The drawing under review shows one solid part. Ordinate dimensions are in mm from its lowest x, y, z. A direction names the side the tool comes from. Coordinates: 2 decimals unless noted, no trailing zeros. Write each loop counter-clockwise with the first axis right and the second up, starting at its lowest first coordinate (ties: lowest second). Pieces come first, ordered by that corner, then holes.
Q1. Machinability: for the marked faces 1, 2 and 3, which of the approach directions +Z, -Z, +X, -X, +Y, -Y give a long, thin tool a straight path to every point of the face, cutting with its end or side? Answer none if there is none.
Q2. Mouldability with a two-part tool opening along Z and no side actions: class the marked faces 4, 5, 6 and 7 as pulls with the +Z half, pulls with the -Z half, needs draft (parallel to the pull), parting line crosses it, or undercut.
Q3. For probe 1 along Z at (x, y) = (825, 170); probe 2 along Z at (x, y) = (845, 150.5); probe 3 along Z at (x, y) = (438, 390.5), list the stretches that pass through material, from the lowest coordinate up.
Q4. Take a section at A-A (y = 136.5). Give the boundary of the cut face in (x, z), and give its area (3 significant figures).
Q5. Insertion check: pin 1 (1 mm diameter, centred on y = 300, z = 417, fed in from +X); pin 2 (12 mm diameter, centred on y = 62.5, z = 791.5, fed in from +X) (1 decimal); pin 3 (10 mm diameter, centred on y = 73.5, z = 890.5, fed in from +X). Each pin has a flat end and moves straight along its axis. Give the tip position at first contact, or say it passes through.
Q6. Take a section at C-C (z = 243.5). Give the boundary of the cut face in (x, y) (1 decimal).
Q7. Take a section at B-B (x = 825.5). Give the boundary of the cut face in (y, z).
Q8. Take a section at D-D (x = 1266). Give the boundary of the cut face in (y, z).
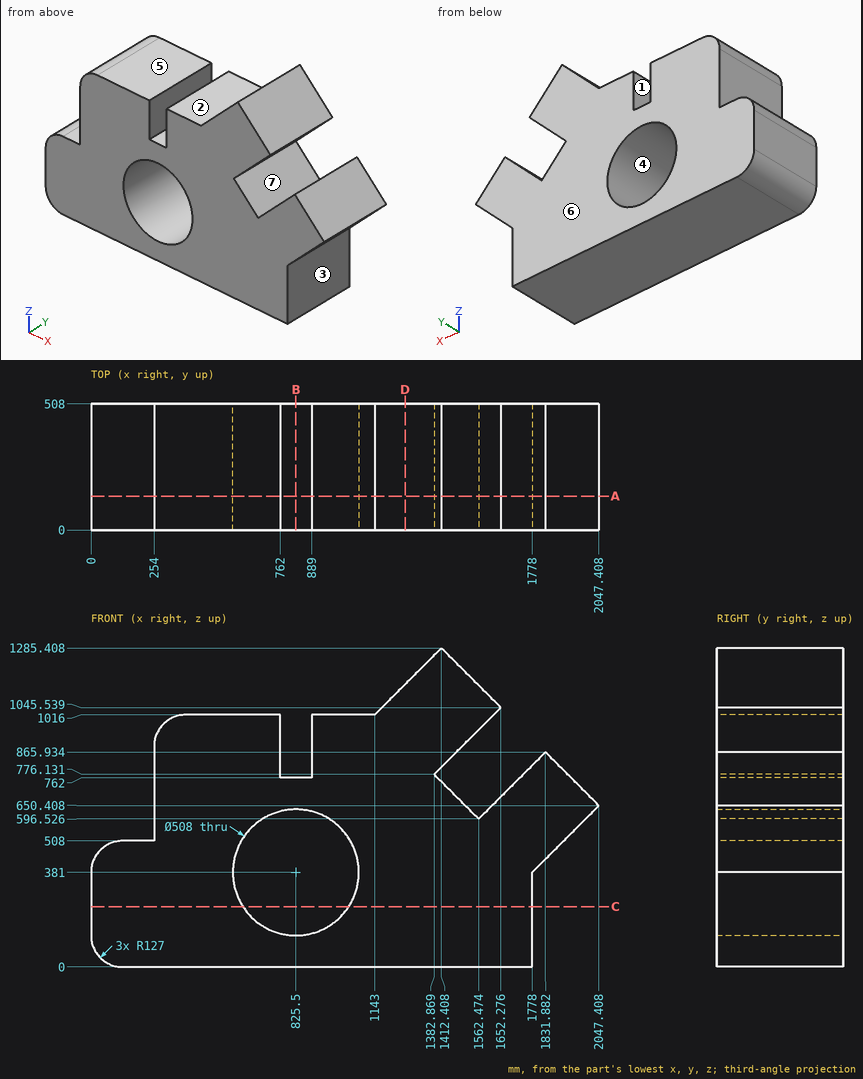
Response:
1. face 1: +Z, +Y, -Y
1. face 2: +Z, -X, +Y, -Y
1. face 3: -Z, +X, +Y, -Y
2. face 4: undercut
2. face 5: pulls with the +Z half
2. face 6: needs draft
2. face 7: undercut
3. probe 1: z = 0 to 127, 635 to 762
3. probe 2: z = 0 to 127.75, 634.25 to 762
3. probe 3: z = 0 to 1016
4. outline: (0, 127) arc R127 ccw to (127, 0) - (1778, 0) - (1778, 381) - (2047.41, 650.41) - (1831.88, 865.93) - (1562.47, 596.53) - (1382.87, 776.13) - (1652.28, 1045.54) - (1412.41, 1285.41) - (1143, 1016) - (889, 1016) - (889, 762) - (762, 762) - (762, 1016) - (381, 1016) arc R127 ccw to (254, 889) - (254, 508) - (127, 508) arc R127 ccw to (0, 381) - close; hole circle Ø508 at (825.5, 381)
4. area: 1,480,000 mm2
5. pin 1: stops at x = 1814.5
5. pin 2: stops at x = 1912.3
5. pin 3: stops at x = 1502.24
6. outline: (0, 0) - (611.9, 0) - (611.9, 508) - (0, 508) - close; (1039.1, 0) - (1778, 0) - (1778, 508) - (1039.1, 508) - close
7. outline: (0, 0) - (508, 0) - (508, 127) - (0, 127) - close; (0, 635) - (508, 635) - (508, 762) - (0, 762) - close
8. outline: (0, 0) - (508, 0) - (508, 1139) - (0, 1139) - close
